from build123d import *

# Parameters (mm, degrees)
F0_R      = 3.175
F1_DEPTH  = 3.81
F3_DEPTH  = 30.48
F2_W      = 50.8
F2_H      = 69.85
F4_DEPTH  = 12.7
F2_W_2    = 19.05
F2_H_2    = 20.32
F5_DEPTH  = 5.08
F2_W_3    = 15.24
F2_H_3    = 38.1
F6_DEPTH  = 7.62
F2_W_4    = 12.7
F7_DEPTH  = 5.08
F8_W      = 16.51
F8_H      = 16.51
F9_DEPTH  = 5.08
F10_W     = 7.62
F10_H     = 2.54
F11_DEPTH = 2.54
F12_W     = 7.62
F12_H     = 12.7
F12_H_2   = 50.8
F13_DEPTH = 5.08
F14_W     = 6.35
F14_H     = 3.679095
F15_DEPTH = 5.08
F16_W     = 12.7
F16_H     = 12.7
F17_DEPTH = 2.54
F18_W     = 7.62
F18_H     = 5.08
F19_DEPTH = 2.54


with BuildPart() as f1:
    # F0 (on Top) → F1 (new body)
    with BuildSketch(Plane.XY):
        with BuildLine():
            Line((98.080416, 92.946989), (-98.769584, 92.946989))
            ThreePointArc((-98.769584, 92.946989), (-100.565635, 92.20304), (-101.309584, 90.406989))
            Line((-101.309584, 90.406989), (-101.309584, -77.233011))
            ThreePointArc((-101.309584, -77.233011), (-100.565635, -79.029062), (-98.769584, -79.773011))
            Line((-98.769584, -79.773011), (98.080416, -79.773011))
            ThreePointArc((98.080416, -79.773011), (99.876467, -79.029062), (100.620416, -77.233011))
            Line((100.620416, -77.233011), (100.620416, 90.406989))
            ThreePointArc((100.620416, 90.406989), (99.876467, 92.20304), (98.080416, 92.946989))
        make_face()
        with Locations((-91.149584, -69.613011)):
            Circle(F0_R, mode=Mode.SUBTRACT)
        with Locations((90.460416, -69.613011)):
            Circle(F0_R, mode=Mode.SUBTRACT)
        with Locations((-91.149584, 82.786989)):
            Circle(F0_R, mode=Mode.SUBTRACT)
        with Locations((90.460416, 82.786989)):
            Circle(F0_R, mode=Mode.SUBTRACT)
    extrude(amount=F1_DEPTH)

    # F2 (on face) → F3 (join)
    with BuildSketch(Plane.XY.offset(3.81)):
        Polygon((-12.409584, 67.546989), (-88.609584, 67.546989), (-88.609584, -28.973011), (-60.669584, -28.973011), (-60.669584, -34.053011), (-12.409584, -34.053011), align=None)
    extrude(amount=F3_DEPTH)

    # F2 (on face) → F4 (join)
    with BuildSketch(Plane.XY.offset(3.81)):
        with Locations((24.420416, -6.748011)):
            Rectangle(F2_W, F2_H)
    extrude(amount=F4_DEPTH)

    # F2 (on face) → F5 (join)
    with BuildSketch(Plane.XY.offset(3.81)):
        with Locations((40.295416, 45.956989)):
            Rectangle(F2_W_2, F2_H_2)
    extrude(amount=F5_DEPTH)

    # F2 (on face) → F6 (join)
    with BuildSketch(Plane.XY.offset(3.81)):
        with Locations((20.610416, 54.846989)):
            Rectangle(F2_W_3, F2_H_3)
    extrude(amount=F6_DEPTH)

    # F2 (on face) → F7 (join)
    with BuildSketch(Plane.XY.offset(3.81)):
        with Locations((4.100416, 54.846989)):
            Rectangle(F2_W_4, F2_H_3)
    extrude(amount=F7_DEPTH)

    # F8 (on face) → F9 (join)
    with BuildSketch(Plane.XZ.offset(34.053011)):
        with Locations((-49.874584, 23.495)):
            Rectangle(F8_W, F8_H)
    extrude(amount=F9_DEPTH)

    # F10 (on face) → F11 (join)
    with BuildSketch(Plane(origin=(0, 67.546989, 0), x_dir=(-1, 0, 0), z_dir=(0, 1, 0))):
        with Locations((77.179584, 15.24)):
            Rectangle(F10_W, F10_H)
    extrude(amount=F11_DEPTH)

    # F12 (on face) → F13 (join)
    with BuildSketch(Plane.XY.offset(16.51)):
        with Locations((46.010416, 21.826989)):
            Rectangle(F12_W, F12_H)
        with Locations((2.830416, 2.776989)):
            Rectangle(F12_W, F12_H_2)
    extrude(amount=F13_DEPTH)

    # F14 (on face) → F15 (join)
    with BuildSketch(Plane.XY.offset(16.51)):
        with Locations((46.645416, -27.133463)):
            Rectangle(F14_W, F14_H)
    extrude(amount=F15_DEPTH)

    # F16 (on face) → F17 (cut)
    with BuildSketch(Plane.XY.offset(16.51)):
        with Locations((30.770416, -35.323011)):
            Rectangle(F16_W, F16_H)
    extrude(amount=-F17_DEPTH, mode=Mode.SUBTRACT)

    # F18 (on face) → F19 (cut)
    with BuildSketch(Plane.XY.offset(16.51)):
        with Locations((15.530416, -39.133011)):
            Rectangle(F18_W, F18_H)
    extrude(amount=-F19_DEPTH, mode=Mode.SUBTRACT)


solid = f1.part
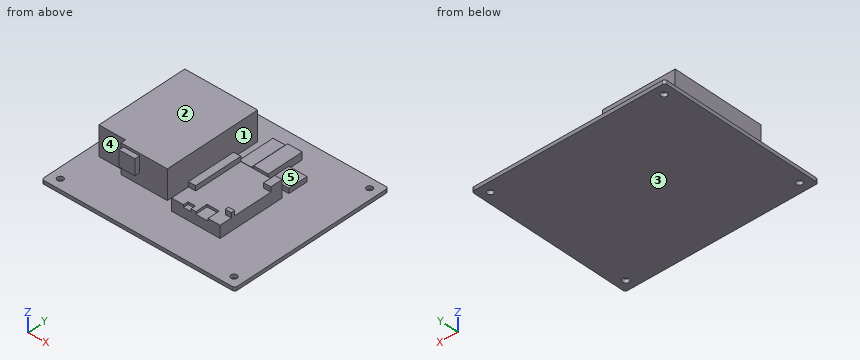
Check sheet for the modelled part. Datum: model origin and axes. Units: mm. Face numbers are marked on the shaded views. A direction names the side the tool comes from. Round coordinates to 2 decimals unless told otherwise and drop trailing zeros. Write each loop counter-clockwise with the first axis right and the second up, starting at its lowest first coordinate (ties: lowest second). Pieces come first, ordered by that corner, then holes. Notation, with made-up numbers: (25.25, 62) - (62.25, 62) arc R21 cw to (62.25, 73) - close; hole circle Ø3 at (9, 47.25). An arc over 180 degrees is marked (long way). Return JSON: item names as keys, results as strings.
Q1. Cross-section at C-C (x = 46). Record the boundary of the cut face in (y, z), then the cut area to 3 significant figures.
Returned:
{"outline": "(-79.77, 0) - (92.95, 0) - (92.95, 3.81) - (56.12, 3.81) - (56.12, 8.89) - (35.8, 8.89) - (35.8, 3.81) - (28.18, 3.81) - (28.18, 21.59) - (15.48, 21.59) - (15.48, 16.51) - (-25.29, 16.51) - (-25.29, 21.59) - (-28.97, 21.59) - (-28.97, 16.51) - (-41.67, 16.51) - (-41.67, 3.81) - (-79.77, 3.81) - close", "area": "1,730 mm²"}
Q2. Cross-section at B-B (y = -17). Record the boundary of the cut face in (x, z).
Returned:
{"outline": "(-101.31, 0) - (100.62, 0) - (100.62, 3.81) - (49.82, 3.81) - (49.82, 16.51) - (6.64, 16.51) - (6.64, 21.59) - (-0.98, 21.59) - (-0.98, 3.81) - (-12.41, 3.81) - (-12.41, 34.29) - (-88.61, 34.29) - (-88.61, 3.81) - (-101.31, 3.81) - close"}
Q3. Cross-section at D-D (z = 24). Record the boundary of the cut face in (x, y), then the cut area to 3 significant figures.
Returned:
{"outline": "(-88.61, -28.97) - (-60.67, -28.97) - (-60.67, -34.05) - (-58.13, -34.05) - (-58.13, -39.13) - (-41.62, -39.13) - (-41.62, -34.05) - (-12.41, -34.05) - (-12.41, 67.55) - (-88.61, 67.55) - close", "area": "7,680 mm²"}
Q4. Scan lines: L1, parallel to X at y = -13, z = 19; L2, parallel to X at y = -8, z = 13; L3, parallel to Z at x = 37, y = 41.5. Record each from-to range of solid material in increasing order. Write a range as from..to.
Returned:
{"L1": "x = -88.61..-12.41, -0.98..6.64", "L2": "x = -88.61..-12.41, -0.98..49.82", "L3": "z = 0..8.89"}
Q5. Depth check by flat-ended pin: P1, Ø1.1, axis at x = 47, y = -28, coming from the +Z side; P2, Ø6, axis at y = 24, z = 15.5, coming from the +X side; P3, Ø15, axis at x = 36.5, y = -14, coming from the +Z side. Enter the tip coordinate at first touch or a pass-through.
Returned:
{"P1": "stops at z = 21.59", "P2": "stops at x = 49.82", "P3": "stops at z = 16.51"}
Q6. Draft check along X on the marked faces 1 and 2. Enter one of: released by +X, released by -X, zero draft, split by the parting line, or undercut.
Returned:
{"face 1": "undercut", "face 2": "zero draft"}
Q7. Access from +Z, -Z, +X, -X, +Y, -Y to the whole of each face (thin tool, end or side, straight path). Record for the marked faces 3, 4 and 5.
Returned:
{"face 3": "-Z, +X, -X, +Y, -Y", "face 4": "+Z, -X, -Y", "face 5": "+Z, +X, +Y"}
Q8. Cross-section at A-A (z = 6). Record the boundary of the cut face in (x, y), then the cut area to 3 significant figures.
Returned:
{"outline": "(-88.61, -28.97) - (-60.67, -28.97) - (-60.67, -34.05) - (-12.41, -34.05) - (-12.41, 67.55) - (-88.61, 67.55) - close; (-2.25, 35.8) - (10.45, 35.8) - (10.45, 73.9) - (-2.25, 73.9) - close; (-0.98, -41.67) - (49.82, -41.67) - (49.82, 28.18) - (-0.98, 28.18) - close; (12.99, 35.8) - (28.23, 35.8) - (28.23, 73.9) - (12.99, 73.9) - close; (30.77, 35.8) - (49.82, 35.8) - (49.82, 56.12) - (30.77, 56.12) - close", "area": "12,600 mm²"}
